Build history of the part. All positions in model axes, mm. A direction names the side the tool comes from. Give positions to 0.01 mm unless a question says otherwise; leave off trailing zeros. Write each loop counter-clockwise with the first axis right and the second up, starting at its lowest first coordinate (ties: lowest second). Pieces come first, ordered by that corner, then holes. Notation, with made-up numbers: (37, -29.75) -> (52, -29.75) arc R20 ccw to (52, -1.75) -> close; hole circle Ø10 at (-27.75, 51). An arc over 180 degrees is marked (long way). Put each result on its own line as item: value. Start each with the question number.
Item 1: Drill centre lines: line 1 along X through (y, z) = (11, -18); line 2 along Z through (x, y) = (-22.6, -7); line 3 along Y through (x, z) = (-22.5, 11.5). Where is each one in solid material? Low to high.
Item 2: Two-plate mould, pull along X, no slides. Class faces 1 (the cylindrical face through (32, 21, 16)), 2 (the cylindrical face through (21.578, 12.054, 17.535)): pulls with the +X half, pulls with the -X half, needs draft (parallel to the pull), parting line crosses it, or undercut.
Item 3: Slice it at D-D, the plane x = -25.5. List the corners of the cut face in (y, z), plus the area to 3 significant figures.
Item 4: Tool access for faces 3 (the flat face through (-17, 17, -18)), 4 (the flat face through (-33, 23.375, 19)), 5 (the flat face through (25, 11, -15)), 6 (the flat face through (-15, -10, 0)), 7 (the flat face through (32, 23.375, -19)): list every direction of +Z, -Z, +X, -X, +Y, -Y with a clear straight run to the whole face (end or side of a thin tool).
Item 5: Flat gauge pins, fed straight in: pin 1 Ø1 at (x, y) = (18, 11.5) entering from -Z; pin 2 Ø5.5 at (x, z) = (26, 17) entering from +Y; pin 3 Ø6 at (y, z) = (-13, 9.5) entering from +X; pin 4 Ø10 at (x, z) = (9.5, 6.5) entering from -Y. Where does each tip first touch, or does it go through?
Item 6: Slice it at B-B, the plane x = -5.25. List the corners of the cut face in (y, z), plus the area to 3 significant figures.
Item 7: Slice it at A-A, the plane y = -11.5. List the corners of the cut face in (x, z).
Item 8: Slice it at C-C, the plane z = -12.5. List the corners of the cut face in (x, y) (3 decimals).
```python
from build123d import *

# Parameters (mm, degrees)
SKETCH1_W               = 70
SKETCH1_H               = 40
BOSS_EXTRUDE1_DEPTH     = 5
BOSS_EXTRUDE2_DEPTH     = 12
SKETCH3_W               = 5
SKETCH3_H               = 40
BOSS_EXTRUDE3_DEPTH     = 10
SKETCH5_R               = 2
CUT_EXTRUDE1_DEPTH      = 78.646635471
CUT_EXTRUDE3_DEPTH      = 57.382621436
CUT_EXTRUDE3_DEPTH_BACK = 57.382621436
SKETCH7_R               = 1.25
SKETCH8_W               = 10
SKETCH8_H               = 0.75
CUT_EXTRUDE4_DEPTH      = 78.646635471
SKETCH9_W               = 4
SKETCH9_H               = 40
BOSS_EXTRUDE4_DEPTH     = 20
CUT_EXTRUDE5_DEPTH      = 50.727549083
CUT_EXTRUDE5_DEPTH_BACK = 50.727549083
SKETCH11_R              = 1.25


with BuildPart() as part:
    # Sketch1 → Boss-Extrude1 (new body)
    with BuildSketch(Plane(origin=(0, 0, 0), x_dir=(1, 0, 0), z_dir=(0, 1, 0))):
        Rectangle(SKETCH1_W, SKETCH1_H)
    extrude(amount=BOSS_EXTRUDE1_DEPTH)

    # Sketch2 → Boss-Extrude2 (add)
    with BuildSketch(Plane(origin=(0, 5, 0), x_dir=(1, 0, 0), z_dir=(0, 1, 0))):
        Polygon((-3, -20), (-3, -15), (-30, -15), (-30, 15), (-3, 15), (-3, 20), (-35, 20), (-35, -20), align=None)
        Polygon((20, -15), (30, -15), (30, 15), (20, 15), (20, 20), (35, 20), (35, -20), (20, -20), align=None)
    extrude(amount=BOSS_EXTRUDE2_DEPTH)

    # Sketch3 → Boss-Extrude3 (add)
    with BuildSketch(Plane(origin=(0, 17, 0), x_dir=(1, 0, 0), z_dir=(0, 1, 0))):
        with Locations((32.5, 0)):
            Rectangle(SKETCH3_W, SKETCH3_H)
        with Locations((-32.5, 0)):
            Rectangle(SKETCH3_W, SKETCH3_H)
    extrude(amount=BOSS_EXTRUDE3_DEPTH)

    # Sketch5 → Cut-Extrude1 (cut, through all)
    with BuildSketch(Plane.ZY.offset(35)):
        with Locations((16, 23)):
            Circle(SKETCH5_R)
        with Locations(Location((-16, 23, 0), (0, 0, 180))):
            Circle(SKETCH5_R)
    extrude(amount=-CUT_EXTRUDE1_DEPTH, mode=Mode.SUBTRACT)

    # Sketch7 → Cut-Extrude3 (cut, two sides: drawn at the far end of the back side and taken through both)
    with BuildSketch(Plane(origin=(0, 0, 15), x_dir=(-1, 0, 0), z_dir=(0, 0, -1)).offset(-CUT_EXTRUDE3_DEPTH_BACK)):
        with Locations((-22.25, 11)):
            Circle(SKETCH7_R)
        with Locations((5.25, 11)):
            Circle(SKETCH7_R)
    extrude(amount=CUT_EXTRUDE3_DEPTH + CUT_EXTRUDE3_DEPTH_BACK, mode=Mode.SUBTRACT)

    # Sketch8 → Cut-Extrude4 (cut, through all)
    with BuildSketch(Plane.ZY.offset(35)):
        with Locations((15, 23)):
            Rectangle(SKETCH8_W, SKETCH8_H)
        with Locations((-15, 23)):
            Rectangle(SKETCH8_W, SKETCH8_H)
    extrude(amount=-CUT_EXTRUDE4_DEPTH, mode=Mode.SUBTRACT)

    # Sketch9 → Boss-Extrude4 (add)
    with BuildSketch(Plane(origin=(0, 0, 0), x_dir=(-1, 0, 0), z_dir=(0, -1, 0))):
        with Locations((21.5, 0)):
            Rectangle(SKETCH9_W, SKETCH9_H)
        with Locations((13, 0)):
            Rectangle(SKETCH9_W, SKETCH9_H)
    extrude(amount=BOSS_EXTRUDE4_DEPTH)

    # Sketch11 → Cut-Extrude5 (cut, two sides: drawn at the far end of the back side and taken through both)
    with BuildSketch(Plane.ZY.offset(1.658275161).offset(-CUT_EXTRUDE5_DEPTH_BACK)):
        with Locations((11.5, -14.5)):
            Circle(SKETCH11_R)
        with Locations((-16, -14.5)):
            Circle(SKETCH11_R)
        with Locations((-16, -7)):
            Circle(SKETCH11_R)
        with Locations((11.5, -7)):
            Circle(SKETCH11_R)
    extrude(amount=CUT_EXTRUDE5_DEPTH + CUT_EXTRUDE5_DEPTH_BACK, mode=Mode.SUBTRACT)


solid = part.part
```
Values follow:
1. line 1: -35 to -6.5, -4 to -3, 20 to 21, 23.5 to 35
1. line 2: -20 to -17.25, -14.75 to 10.25, 12.75 to 20
1. line 3: -20 to -15.75, -13.25 to -8.25, -5.75 to 5
2. face 1: needs draft
2. face 2: undercut
3. outline: (0, -20) -> (17, -20) -> (17, -15) -> (5, -15) -> (5, 15) -> (17, 15) -> (17, 20) -> (0, 20) -> close
3. area: 320 mm2
4. face 3: +Z, -Z, +Y
4. face 4: +Z, +X, -X
4. face 5: +Y
4. face 6: +Z, -Z, -Y
4. face 7: -Z, +X, -X
5. pin 1: through
5. pin 2: y = 17
5. pin 3: x = -11
5. pin 4: y = 0
6. outline: (0, -20) -> (9.75, -20) -> (9.75, -15) -> (5, -15) -> (5, 15) -> (9.75, 15) -> (9.75, 20) -> (0, 20) -> close; (12.25, -20) -> (17, -20) -> (17, -15) -> (12.25, -15) -> close; (12.25, 15) -> (17, 15) -> (17, 20) -> (12.25, 20) -> close
6. area: 295 mm2
7. outline: (-23.5, -20) -> (-19.5, -20) -> (-19.5, 20) -> (-23.5, 20) -> close; (-15, -20) -> (-11, -20) -> (-11, 20) -> (-15, 20) -> close
8. outline: (-35, 0) -> (-23.5, 0) -> (-23.5, -20) -> (-19.5, -20) -> (-19.5, 0) -> (-15, 0) -> (-15, -20) -> (-11, -20) -> (-11, 0) -> (35, 0) -> (35, 22.625) -> (30, 22.625) -> (30, 5) -> (-30, 5) -> (-30, 22.625) -> (-35, 22.625) -> close; (-35, 23.375) -> (-30, 23.375) -> (-30, 27) -> (-35, 27) -> close; (30, 23.375) -> (35, 23.375) -> (35, 27) -> (30, 27) -> close
